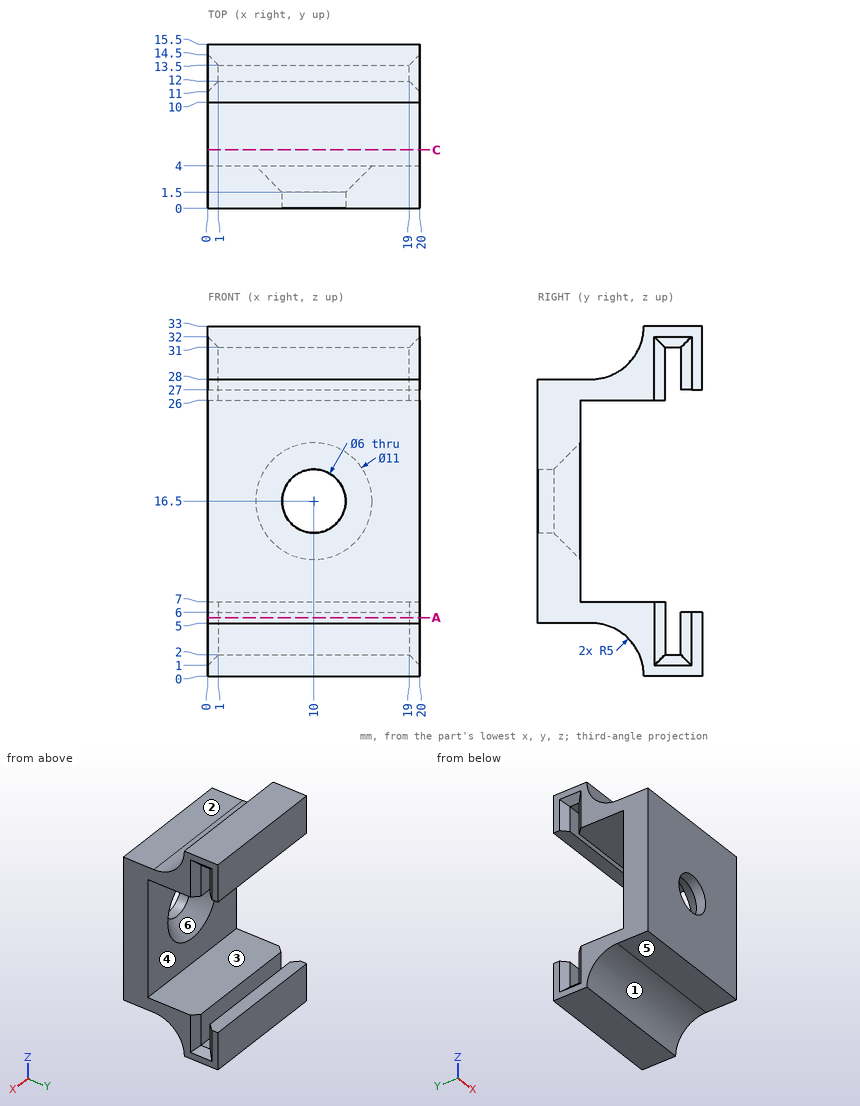
The drawing under review shows one solid part. Ordinate dimensions are in mm from its lowest x, y, z. A direction names the side the tool comes from. Coordinates: 2 decimals unless noted, no trailing zeros. Write each loop counter-clockwise with the first axis right and the second up, starting at its lowest first coordinate (ties: lowest second). Pieces come first, ordered by that corner, then holes.
1) Machinability: for the marked faces 4, 5 and 6, which of the approach directions +Z, -Z, +X, -X, +Y, -Y give a long, thin tool a straight path to every point of the face, cutting with its end or side? Answer none if there is none.
2) To check wall thickness, follow L1, parallel to Z at x = 10, y = 0.7; L2, parallel to X at y = 0.8, z = 16.5; L3, parallel to Z at x = 18, y = 4.25. State the ranges of each line that lie inside material, in increasing order.
3) Insertion check: pin 1 (5.5 mm diameter, centred on x = 8, y = 2.5, fed in from +Z); pin 2 (4 mm diameter, centred on x = 13.5, y = 6, fed in from -Z); pin 3 (2.5 mm diameter, centred on x = 9, y = 3.5, fed in from -Z). Each pin has a flat end and moves straight along its axis. Give the tip position at first contact, or say it passes through.
4) Mouldability with a two-part tool opening along Z and no side actions: class the marked faces 1, 2 and 3 as +Z half, -Z half, draft (parallel to the pull), parting line (faces both ways), or undercut.
5) Add section C-C (y = 5.5). Write out the cut boundary in (x, z) (1 decimal).
6) Add section A-A (z = 5.5). Write out the cut boundary in (x, y).
Check result:
1. face 4: +X, -X, +Y
1. face 5: -Z, +X, -X, -Y
1. face 6: +Y
2. L1: z = 5 to 13.5, 19.5 to 28
2. L2: x = 0 to 7, 13 to 20
2. L3: z = 5 to 7, 26 to 28
3. pin 1: stops at z = 28.01
3. pin 2: stops at z = 4
3. pin 3: stops at z = 5
4. face 1: -Z half
4. face 2: +Z half
4. face 3: undercut
5. outline: (0, 5) - (20, 5) - (20, 7) - (0, 7) - close; (0, 26) - (20, 26) - (20, 28) - (0, 28) - close
6. outline: (0, 0) - (20, 0) - (20, 11) - (19, 12) - (1, 12) - (0, 11) - close; (0, 14.5) - (1, 13.5) - (19, 13.5) - (20, 14.5) - (20, 15.5) - (0, 15.5) - close
